Can you work these out from the model? Positions are in its coordinate system, mm. A direction names the side the tool comes from. Give positions to 0.01 mm unless a question says otherwise; leave off trailing zeros. Loops run counter-clockwise (first coordinate to the right, second up) from the corner with the lowest first, then second, coordinate; pieces in that order, holes last. Notation, with made-up numbers: (21.5, 67) -> (44.5, 67) arc R29 ccw to (44.5, 92) -> close; hole circle Ø7 at (63, 33.5). An arc over 180 degrees is marked (long way). Return JSON: item names as keys, results as strings. Group by question number.
Q1. Which directions (+Z, -Z, +X, -X, +Y, -Y) give clear straight access to the entire face, cutting with the end or side of a thin tool? Please do faces 4 (the flat face through (-2, 1, 13)), 5 (the flat face through (-1, -2, 22.5)), 6 (the flat face through (1.5, 3, -4)), 7 (the cylindrical face through (-0.09, -1.46, -12.35)), 8 (the flat face through (-3.39, -2.67, 13)).
Q2. Suppose I cut it at D-D, the plane z = -1.5. Please give me the cut outline in (x, y).
Q3. Suppose I cut it at C-C, the plane y = -2.5. Please give me the cut outline in (x, z) (1 decimal), and give its area (3 significant figures).
Q4. Thinking about a two-plate mould opening in X: for faces 1 (the flat face through (-10.5, -4, 0)), 2 (the flat face through (-9, -9, 0)), 3 (the flat face through (1, 3, -7)), which applies, pulls with the +X half, pulls with the -X half, needs draft (parallel to the pull), parting line crosses it, or undercut?
Q5. Suppose I cut it at B-B, the plane z = -14.5. Please give me the cut outline in (x, y).
Q6. I need wall thicknesses on line 1 along Z through (x, y) = (0, 0.3); line 2 along Z through (x, y) = (0, 3.15); line 3 along X through (y, z) = (0.25, 15). Which ranges of each line are inside material? Lowest first, please. Write a range as [from, to].
Q7. Will these pins go through, and if not, where does the flat tip stop? pin 1 (1 mm diameter, centred on x = -6.5, z = -4, fed in from +Y); pin 2 (1 mm diameter, centred on x = 0, y = 2.5, fed in from +Z); pin 3 (5 mm diameter, centred on x = -7, z = 11, fed in from -Y); pin 4 (2 mm diameter, centred on x = -5, z = -3.5, fed in from -Y).
Q8. Suppose I cut it at A-A, the plane x = 0. Please give me the cut outline in (y, z), and give its area (3 significant figures).
Autodesk Inventor part; units mm, degrees
ref_plane "YZ Plane" through (0, 0, 0) normal (1, 0, 0) x (0, 1, 0)
ref_plane "XZ Plane" through (0, 0, 0) normal (0, 1, 0) x (-1, 0, 0)
ref_plane "XY Plane" through (0, 0, 0) normal (0, 0, 1) x (1, 0, 0)
sketch "Sketch1" plane through (0, 0, 0) normal (0, 1, 0) x (-1, 0, 0)
  line L0 (-7.5, 22.5) -> (10.5, 22.5)
  line L1 (10.5, 22.5) -> (10.5, -22.5)
  line L2 (10.5, -22.5) -> (-7.5, -22.5)
  line L3 (-7.5, -22.5) -> (-7.5, 22.5)
  point P0 (0, 0)
  point P1 (-7.5, 0)
  dimension "d0" = 45
  dimension "d1" = 18
  dimension "d97" = 7.5
extrude "Extrusion1" add sketch "Sketch1" along normal mid plane 8
sketch "Sketch4" plane through (0, 4, 0) normal (0, 1, 0) x (1, 0, 0)
  line L0 (-10.5, -7.5) -> (7.5, -7.5)
  line L1 (7.5, -7.5) -> (7.5, -5.5)
  line L2 (7.5, -5.5) -> (-10.5, -5.5)
  line L3 (-10.5, -5.5) -> (-10.5, -7.5)
  line L4 (-10.5, -22.5) -> (7.5, -22.5)
  line L5 (-10.5, 22.5) -> (-10.5, -22.5)
  line L6 (7.5, -22.5) -> (7.5, 22.5)
  dimension "d57" = 2
  dimension "d58" = 15
extrude "Extrusion3" add sketch "Sketch4" along normal blind 5 contours L3 L2 L1 L0
sketch "Sketch5" plane through (0, 4, 0) normal (0, 1, 0) x (1, 0, 0)
  line L0 (-7.5, 7) -> (-5.5, 7)
  line L1 (-5.5, 7) -> (-5.5, 1)
  line L2 (-5.5, 1) -> (-7.5, 1)
  line L3 (-7.5, 1) -> (-7.5, 7)
  line L4 (1.5, 7) -> (-0.5, 7)
  line L5 (-0.5, 7) -> (-0.5, 1)
  line L6 (-0.5, 1) -> (1.5, 1)
  line L7 (1.5, 1) -> (1.5, 7)
  line L8 (-6.5, 4) -> (0.5, 4) construction
  line L9 (7.5, -5.5) -> (-7.5, -5.5) construction
  line L10 (-7.5, 7.8654) -> (-7.5, -0.5) construction
  line L11 (-7.5, -0.5) -> (-22.5, -0.5) construction
  line L12 (7.5, -5.5) -> (-10.5, -5.5)
  line L13 (7.5, 22.5) -> (-10.5, 22.5)
  line L14 (-10.5, 22.5) -> (-10.5, -5.5)
  point P0 (0, -5.5)
  point P1 (0.5, 7)
  point P2 (-6.5, 7)
  point P3 (-5.5, 4)
  point P4 (0, 0)
  point P5 (-3, 4)
  point P6 (-1.5, 22.5)
  dimension "d20" = 6
  dimension "d21" = 2
  dimension "d22" = 5
  dimension "d26" = 1.5
  dimension "d31" = 7
  dimension "d103" = 7.5
extrude "Extrusion4" cut sketch "Sketch5" against normal blind 3
sketch "Sketch7" plane through (-10.5, -4, -12.5) normal (-1, 0, 0) x (0, 0, 1)
  line L0 (20, 8) -> (35, 8)
  line L1 (20, 8) -> (35, 8)
  line L2 (35, 8) -> (35, 5)
  line L3 (35, 5) -> (20, 5)
  line L4 (20, 5) -> (20, 8)
  line L5 (35, 8) -> (35, 0)
  point P0 (12.5, 4)
  dimension "d59" = 3
extrude "Extrusion6" cut sketch "Sketch7" against normal through all
sketch "Sketch8" plane through (0, 4, 0) normal (0, 1, 0) x (1, 0, 0)
  line L0 (-10.5, -5.5) -> (-10, -5.5)
  line L1 (-10, -5.5) -> (-10, -3.5)
  line L2 (-10, -3.5) -> (-10.5, -3.5)
  line L3 (-10.5, -3.5) -> (-10.5, -5.5)
  dimension "d60" = 2
  dimension "d61" = 0.5
extrude "Extrusion7" add sketch "Sketch8" along normal blind 1
sketch "Sketch13" plane through (-10.5, 1, 22.5) normal (0, 1, 0) x (1, 0, 0)
  line L0 (18, 15) -> (18, 0)
  point P0 (10.5, 22.5)
  point P1 (10.5, 7.5)
  point P2 (18, 7.5)
hole "Hole3" at (0, 1, 15) direction (0, -1, 0) diameter 3.797 end through all
sketch "Sketch12" plane through (0, -4, 0) normal (0, -1, 0) x (1, 0, 0)
  line L0 (7.5, 22.5) -> (-10.5, 22.5)
  line L1 (-2.273, 11.063) -> (-4.5461, 15)
  line L2 (-4.5461, 15) -> (-2.273, 18.937)
  line L3 (-2.273, 18.937) -> (2.273, 18.937)
  line L4 (2.273, 18.937) -> (4.5461, 15)
  line L5 (4.5461, 15) -> (2.273, 11.063)
  line L6 (2.273, 11.063) -> (-2.273, 11.063)
  circle A0 centre (0, 15) radius 1.8985
  point P0 (0, 0)
  dimension "d98" = 7.874
extrude "Extrusion10" cut sketch "Sketch12" against normal blind 2.7
sketch "Sketch14" plane through (0, 4, 0) normal (0, 1, 0) x (1, 0, 0)
  circle A0 centre (0, 14.5) radius 3.81
  line L0 (7.5, 22.5) -> (-10.5, 22.5)
  point P0 (0, 0)
  dimension "d95" = 7.62
  dimension "d96" = 8
extrude "Extrusion11" cut sketch "Sketch14" against normal blind 3
sketch "Sketch15" plane through (0, -4, 0) normal (0, -1, 0) x (1, 0, 0)
  line L0 (-10.5, -22.5) -> (7.5, -22.5)
  point P0 (0, 0)
  point P1 (0, -14.5)
  dimension "d87" = 8
hole "Hole4" at (0, -4, -14.5) direction (0, 1, 0) diameter 4.305 end through all
sketch "Sketch16" plane through (0, -4, 0) normal (0, -1, 0) x (1, 0, 0)
  line L0 (7.5, 22.5) -> (-10.5, 22.5)
  line L1 (-10.5, 22.5) -> (-7.5, 22.5)
  line L2 (-7.5, 22.5) -> (-7.5, -22.5)
  line L3 (-7.5, -22.5) -> (-10.5, -22.5)
  line L4 (-10.5, -22.5) -> (-10.5, 22.5)
  line L5 (-10.5, -22.5) -> (7.5, -22.5)
  line L6 (7.5, -22.5) -> (7.5, 22.5)
  point P0 (0, 0)
  dimension "d102" = 15
extrude "Extrusion12" add sketch "Sketch16" along normal blind 5 contours L2 L3 L4 L0
properties part number "FixedFiber"
Ans:
{
 "1": {"face 4": "+Z, +X, -X, +Y", "face 5": "+Z, +X, -X, +Y, -Y", "face 6": "+Y", "face 7": "+Y, -Y", "face 8": "-Y"},
 "2": {"outline": "(-10.5, -9) -> (-7.5, -9) -> (-7.5, -4) -> (7.5, -4) -> (7.5, 4) -> (1.5, 4) -> (1.5, 1) -> (-0.5, 1) -> (-0.5, 4) -> (-5.5, 4) -> (-5.5, 1) -> (-7.5, 1) -> (-7.5, 4) -> (-10.5, 4) -> close"},
 "3": {"outline": "(-10.5, -22.5) -> (7.5, -22.5) -> (7.5, 22.5) -> (-10.5, 22.5) -> close; hole (-4.5, 15) -> (-2.3, 11.1) -> (2.3, 11.1) -> (4.5, 15) -> (2.3, 18.9) -> (-2.3, 18.9) -> close; hole circle Ø4.3 at (0, -14.5)", "area": "742 mm^2"},
 "4": {"face 1": "pulls with the -X half", "face 2": "needs draft", "face 3": "undercut"},
 "5": {"outline": "(-10.5, -9) -> (-7.5, -9) -> (-7.5, -4) -> (-2.15, -4) -> (-2.15, 1) -> (-3.81, 1) -> (-3.81, 4) -> (-10.5, 4) -> close; (2.15, -4) -> (7.5, -4) -> (7.5, 4) -> (3.81, 4) -> (3.81, 1) -> (2.15, 1) -> close"},
 "6": {"line 1": "z = [-22.5, -16.65], [-12.35, 13.1], [16.9, 22.5]", "line 2": "z = [-22.5, -18.31], [-10.69, -7], [-1, 7.5]", "line 3": "x = [-10.5, -1.9], [1.9, 7.5]"},
 "7": {"pin 1": "stops at y = 1", "pin 2": "stops at z = 7.5", "pin 3": "stops at y = -9", "pin 4": "stops at y = -4"},
 "8": {"outline": "(-4, -22.5) -> (4, -22.5) -> (4, -18.31) -> (1, -18.31) -> (1, -16.65) -> (-4, -16.65) -> close; (-4, -12.35) -> (1, -12.35) -> (1, -10.69) -> (4, -10.69) -> (4, -7) -> (1, -7) -> (1, -1) -> (4, -1) -> (4, 5.5) -> (9, 5.5) -> (9, 7.5) -> (1, 7.5) -> (1, 13.1) -> (-1.3, 13.1) -> (-1.3, 11.06) -> (-4, 11.06) -> close; (-4, 18.94) -> (-1.3, 18.94) -> (-1.3, 16.9) -> (1, 16.9) -> (1, 22.5) -> (-4, 22.5) -> close", "area": "233 mm^2"}
}
